```python
from build123d import *

# Parameters (mm, degrees)
CROQUIS1_R              = 17
CROQUIS1_R_2            = 1.5
SALIENTE_EXTRUIR1_DEPTH = 4
CORTAR_EXTRUIR1_DEPTH   = 4
SALIENTE_EXTRUIR2_START = 6
CROQUIS3_R              = 9
CROQUIS3_R_2            = 1.5
SALIENTE_EXTRUIR2_DEPTH = 6


with BuildPart() as part:
    # Croquis1 → Saliente-Extruir1 (new body)
    with BuildSketch(Plane.XY):
        Circle(CROQUIS1_R)
        with Locations((0, 12.5)):
            Circle(CROQUIS1_R_2, mode=Mode.SUBTRACT)
        with Locations((10.825317547, -6.25)):
            Circle(CROQUIS1_R_2, mode=Mode.SUBTRACT)
        with Locations((-10.825317547, -6.25)):
            Circle(CROQUIS1_R_2, mode=Mode.SUBTRACT)
    extrude(amount=SALIENTE_EXTRUIR1_DEPTH)

    # Croquis2 → Cortar-Extruir1 (cut)
    with BuildSketch(Plane(origin=(0, 0, 0), x_dir=(-1, 0, 0), z_dir=(0, 0, -1))):
        Polygon((3.550704156, 6.15), (-3.550704156, 6.15), (-7.101408311, 0), (-3.550704156, -6.15), (3.550704156, -6.15), (7.101408311, 0), align=None)
    extrude(amount=-CORTAR_EXTRUIR1_DEPTH, mode=Mode.SUBTRACT)

    # Croquis3 → Saliente-Extruir2 (add)
    # profile 1 of 4: a face of its own
    with BuildSketch(Plane(origin=(0, 0, 0), x_dir=(-1, 0, 0), z_dir=(0, 0, -1)).offset(SALIENTE_EXTRUIR2_START)):
        Circle(CROQUIS3_R)
        Polygon((-7.101408311, 0), (-3.550704156, 6.15), (3.550704156, 6.15), (7.101408311, 0), (3.550704156, -6.15), (-3.550704156, -6.15), align=None, mode=Mode.SUBTRACT)
    # profile 2 of 4: a face of its own
    with BuildSketch(Plane(origin=(0, 0, 0), x_dir=(-1, 0, 0), z_dir=(0, 0, -1)).offset(SALIENTE_EXTRUIR2_START)):
        with Locations(Location((0, 12.5, 0), (0, 0, 180))):
            Circle(CROQUIS3_R_2)
    # profile 3 of 4: a face of its own
    with BuildSketch(Plane(origin=(0, 0, 0), x_dir=(-1, 0, 0), z_dir=(0, 0, -1)).offset(SALIENTE_EXTRUIR2_START)):
        with Locations(Location((-10.825317547, -6.25, 0), (0, 0, 180))):
            Circle(CROQUIS3_R_2)
    # profile 4 of 4: a face of its own
    with BuildSketch(Plane(origin=(0, 0, 0), x_dir=(-1, 0, 0), z_dir=(0, 0, -1)).offset(SALIENTE_EXTRUIR2_START)):
        with Locations(Location((10.825317547, -6.25, 0), (0, 0, 180))):
            Circle(CROQUIS3_R_2)
    extrude(amount=-SALIENTE_EXTRUIR2_DEPTH)


with BuildPart() as saliente_extruir2_kept_piece:
    # of the separate pieces the step leaves, the one the design keeps (saliente_extruir2_pieces_kept)
    add(part.part.solids().sort_by_distance((17, 0, 0))[0])


solid = saliente_extruir2_kept_piece.part
```
CAD build for the part. Positions are in the model's coordinates, mm. A direction names the side the tool comes from. Coordinates: 2 decimals unless noted, no trailing zeros. Write each loop counter-clockwise with the first axis right and the second up, starting at its lowest first coordinate (ties: lowest second). Pieces come first, ordered by that corner, then holes.
(1) 3-axis set-ups, long thin cutter, end or side, ignore diameter. For faces 1 (the face through (5.3, -3.12, -1.07)), 2 (the face through (7.3, 0.2, 4)): which of +Z, -Z, +X, -X, +Y, -Y reach the whole face in a straight line?
(2) Cut at B-B, the plane y = 12. List the corners of the cut face in (x, z), and give its area (3 significant figures).
(3) Drill centre lines: probe 1 along Y at (x, z) = (0, 1.1); probe 2 along X at (y, z) = (-6, 1.75); probe 3 along X at (y, z) = (3, -1.5). Where is each one in solid material? Low to high.
(4) Cut at D-D, the plane z = -4.25. List the corners of the cut face in (x, y).
(5) Flat gauge pins, fed straight in: pin 1 (3.5 mm diameter, centred on x = 1, z = -3, fed in from +Y); pin 2 (2 mm diameter, centred on x = 5, z = -0.5, fed in from +Y); pin 3 (1.8 mm diameter, centred on x = 0, y = 12.5, fed in from +Z). Where does each tip first touch, or does it go through?
(6) Cut at C-C, the plane z = 3.25. List the corners of the cut face in (x, y), and give its area (3 significant figures).
(7) Two-plate mould, pull along X, no slides. Class faces 3 (the face through (1.172, 8.923, -3.042)), 4 (the face through (7, -7, 0)), 5 (the face through (-9.44, -6.82, 1.97)): +X half, -X half, draft (parallel to the pull), parting line (faces both ways), or undercut.
(8) Cut at A-A, the plane x = 0. List the corners of the cut face in (y, z).
Geometry says:
1. face 1: +Z, -Z
1. face 2: +Z, +X, -X, +Y, -Y
2. outline: (-12.04, 0) - (-1.41, 0) - (-1.41, 4) - (-12.04, 4) - close; (1.41, 0) - (12.04, 0) - (12.04, 4) - (1.41, 4) - close
2. area: 85.0 mm2
3. probe 1: y = -17 to -6.15, 6.15 to 11, 14 to 17
3. probe 2: x = -15.91 to -12.3, -9.35 to -3.64, 3.64 to 9.35, 12.3 to 15.91
3. probe 3: x = -8.49 to -5.37, 5.37 to 8.49
4. outline: circle Ø18 at (0, 0); hole (-7.1, 0) - (-3.55, -6.15) - (3.55, -6.15) - (7.1, 0) - (3.55, 6.15) - (-3.55, 6.15) - close
5. pin 1: stops at y = 9
5. pin 2: stops at y = 16.49
5. pin 3: passes through
6. outline: circle Ø34 at (0, 0); hole circle Ø3 at (-10.83, -6.25); hole (-7.1, 0) - (-3.55, -6.15) - (3.55, -6.15) - (7.1, 0) - (3.55, 6.15) - (-3.55, 6.15) - close; hole circle Ø3 at (0, 12.5); hole circle Ø3 at (10.83, -6.25)
6. area: 756 mm2
7. face 3: parting line
7. face 4: draft
7. face 5: undercut
8. outline: (-17, 0) - (-9, 0) - (-9, -6) - (-6.15, -6) - (-6.15, 4) - (-17, 4) - close; (6.15, -6) - (9, -6) - (9, 0) - (11, 0) - (11, 4) - (6.15, 4) - close; (14, 0) - (17, 0) - (17, 4) - (14, 4) - close
